Check sheet for the modelled part. Datum: model origin and axes. Units: mm. A direction names the side the tool comes from. Coordinates: 2 decimals unless noted, no trailing zeros. Write each loop counter-clockwise with the first axis right and the second up, starting at its lowest first coordinate (ties: lowest second). Pieces come first, ordered by that corner, then holes. Notation, with made-up numbers: M 21,-38 L 77,-38 A27 ccw 77,-5 Z; hole C 80,17 d5. An arc over 180 degrees is marked long. Answer as CSV lines item,"result".
from build123d import *

# Parameters (mm, degrees)
SKETCH8_R           = 14
BOSS_EXTRUDE6_DEPTH = 10
SKETCH9_R           = 2.5
CUT_EXTRUDE1_DEPTH  = 10
CUT_EXTRUDE2_DEPTH  = 10


with BuildPart() as part:
    # Sketch8 → Boss-Extrude6 (new body)
    with BuildSketch(Plane.XY):
        Circle(SKETCH8_R)
    extrude(amount=BOSS_EXTRUDE6_DEPTH)

    # Sketch9 → Cut-Extrude1 (cut)
    with BuildSketch(Plane.XY.offset(10)):
        Circle(SKETCH9_R)
    extrude(amount=-CUT_EXTRUDE1_DEPTH, mode=Mode.SUBTRACT)

    # Sketch10 → Cut-Extrude2 (cut)
    with BuildSketch(Plane.XY.offset(10)):
        with BuildLine():
            ThreePointArc((-4.299671038, -1.327715693), (-3.897114317, 2.25), (-1, 4.387482194))
            Line((-1, 4.387482194), (-1, 11.958260743))
            ThreePointArc((-1, 11.958260743), (-10.392304845, 6), (-10.856157589, -5.113104968))
            Line((-10.856157589, -5.113104968), (-4.299671038, -1.327715693))
        make_face()
        with BuildLine():
            Line((1, 11.958260743), (1, 4.387482194))
            ThreePointArc((1, 4.387482194), (3.51781182, 2.80624304), (4.5, 0))
            ThreePointArc((4.5, 0), (4.449635922, -0.671371852), (4.299671038, -1.327715693))
            Line((4.299671038, -1.327715693), (10.856157589, -5.113104968))
            ThreePointArc((10.856157589, -5.113104968), (11.710548473, -2.619743207), (12, 0))
            ThreePointArc((12, 0), (8.831760866, 8.124038405), (1, 11.958260743))
        make_face()
        with BuildLine():
            ThreePointArc((3.299671038, -3.059766501), (0, -4.5), (-3.299671038, -3.059766501))
            Line((-3.299671038, -3.059766501), (-9.856157589, -6.845155775))
            ThreePointArc((-9.856157589, -6.845155775), (0, -12), (9.856157589, -6.845155775))
            Line((9.856157589, -6.845155775), (3.299671038, -3.059766501))
        make_face()
    extrude(amount=-CUT_EXTRUDE2_DEPTH, mode=Mode.SUBTRACT)


solid = part.part
1) Section check C-C, the plane x = -10.5. Record the boundary of the cut face in (y, z).
Answer key:
outline,"M -9.26,0 L -4.91,0 L -4.91,10 L -9.26,10 Z; M 5.81,0 L 9.26,0 L 9.26,10 L 5.81,10 Z"
2) Tool access check on faces 1 (the face through (-3.923, 2.205, 5.07)), 2 (the face through (0, -3, 10)). Record the directions out of +Z, -Z, +X, -X, +Y, -Y that give a thin tool (end or side, any length) a straight path to the whole face; none if there is none.
Answer key:
face 1,"+Z, -Z"
face 2,"+Z, +X, -X, +Y, -Y"
3) Section check B-B, the plane z = 6. Record the boundary of the cut face in (x, y), plus the area to 3 significant figures.
Answer key:
outline,"C 0,0 d28; hole M -10.86,-5.11 L -4.3,-1.33 A4.5 cw -1,4.39 L -1,11.96 A12 ccw Z; hole M -9.86,-6.85 A12 ccw 9.86,-6.85 L 3.3,-3.06 A4.5 cw -3.3,-3.06 Z; hole C 0,0 d5; hole M 1,4.39 A4.5 cw 4.3,-1.33 L 10.86,-5.11 A12 ccw 1,11.96 Z"
area,"252 mm2"
4) Thickness scan on line 1 along X through (y, z) = (5.75, 5.5); line 2 along Y through (x, z) = (0, 6.75); line 3 along Y through (x, z) = (-1.25, 7.75). Record the ranges inside material, lowest first.
Answer key:
line 1,"x = -12.76 to -10.53, -1 to 1, 10.53 to 12.76"
line 2,"y = -14 to -12, -4.5 to -2.5, 2.5 to 14"
line 3,"y = -13.94 to -11.93, -4.32 to -2.17, 2.17 to 4.32, 11.93 to 13.94"
5) Section check A-A, the plane x = 0. Record the boundary of the cut face in (y, z), plus the area to 3 significant figures.
Answer key:
outline,"M -14,0 L -12,0 L -12,10 L -14,10 Z; M -4.5,0 L -2.5,0 L -2.5,10 L -4.5,10 Z; M 2.5,0 L 14,0 L 14,10 L 2.5,10 Z"
area,"155 mm2"
6) Section check D-D, the plane y = -8.5. Record the boundary of the cut face in (x, z), plus the area to 3 significant figures.
Answer key:
outline,"M -11.12,0 L -8.47,0 L -8.47,10 L -11.12,10 Z; M 8.47,0 L 11.12,0 L 11.12,10 L 8.47,10 Z"
area,"53.1 mm2"
7) Mould release check, pull along X, two halves, no side actions. Record for faces 3 (the face through (-10.31, 6.14, 5.07)), 4 (the face through (6.624, -4.979, 5.07)), 5 (the face through (0, -3, 0)), 6 (the face through (12.932, -5.362, 4.93)): pulls with the +X half, pulls with the -X half, needs draft (parallel to the pull), parting line crosses it, or undercut.
Answer key:
face 3,"undercut"
face 4,"undercut"
face 5,"needs draft"
face 6,"parting line crosses it"
8) Depth check by flat-ended pin: P1, Ø2, axis at y = 8, z = 2.5, coming from the +X side; P2, Ø3, axis at x = 10.5, z = 3.5, coming from the +Y side; P3, Ø2, axis at y = 2.5, z = 6, coming from the -X side. Enter the tip coordinate at first touch or a pass-through.
Answer key:
P1,"stops at x = 12.12"
P2,"stops at y = 10.72"
P3,"stops at x = -13.92"
